Geometry check sheet. Reference: the model listing, model coordinates, mm. A direction names the side the tool comes from. Coordinates: 2 decimals unless noted, no trailing zeros. Loops run counter-clockwise (first coordinate to the right, second up) from the corner with the lowest first, then second, coordinate; pieces in that order, holes last. Notation, with made-up numbers: (17.5, 67) - (62.5, 67) arc R27 cw to (62.5, 95) - close; hole circle Ø1 at (-9.75, 52). An arc over 180 degrees is marked (long way). Write item = value, one per line. Start each with the question number.
from build123d import *

# Parameters (mm, degrees)
SZKIC1_W                    = 27
SZKIC1_H                    = 30
SZKIC1_R                    = 1.6
DODANIE_WYCI_GNI_CIE1_DEPTH = 2
DODANIE_WYCI_GNI_CIE2_DEPTH = 8
ZAOKR_GLENIE1_R             = 4
ZAOKR_GLENIE2_R             = 2


with BuildPart() as part:
    # Szkic1 → Dodanie-wyciągnięcie1 (new body)
    with BuildSketch(Plane(origin=(0, 0, 0), x_dir=(1, 0, 0), z_dir=(0, 1, 0))):
        Rectangle(SZKIC1_W, SZKIC1_H)
        with Locations(Location((10, 0, 0), (0, 0, 270))):
            Circle(SZKIC1_R, mode=Mode.SUBTRACT)
        with Locations(Location((-10, 0, 0), (0, 0, 270))):
            Circle(SZKIC1_R, mode=Mode.SUBTRACT)
    extrude(amount=DODANIE_WYCI_GNI_CIE1_DEPTH)

    # Szkic2 → Dodanie-wyciągnięcie2 (add)
    with BuildSketch(Plane.XZ):
        with BuildLine():
            Line((-13.5, 8), (-13.5, 15))
            Line((-13.5, 15), (-6.5, 15))
            ThreePointArc((-6.5, 15), (-8.550252532, 10.050252532), (-13.5, 8))
        make_face()
        with BuildLine():
            Line((13.5, 8), (13.5, 15))
            Line((13.5, 15), (6.5, 15))
            ThreePointArc((6.5, 15), (8.550252532, 10.050252532), (13.5, 8))
        make_face()
        with BuildLine():
            Line((13.5, -15), (6.5, -15))
            ThreePointArc((6.5, -15), (8.550252532, -10.050252532), (13.5, -8))
            Line((13.5, -8), (13.5, -15))
        make_face()
        with BuildLine():
            Line((-13.5, -8), (-13.5, -15))
            Line((-13.5, -15), (-6.5, -15))
            ThreePointArc((-6.5, -15), (-8.550252532, -10.050252532), (-13.5, -8))
        make_face()
    extrude(amount=DODANIE_WYCI_GNI_CIE2_DEPTH)

    # Zaokrąglenie1
    zaokr_glenie1_edges = [part.edges().sort_by_distance(p)[0] for p in [
        (13.5, -3, 15),
        (-13.5, -3, 15),
        (-13.5, -3, -15),
        (13.5, -3, -15),
    ]]
    fillet(zaokr_glenie1_edges, radius=ZAOKR_GLENIE1_R)

    # Zaokrąglenie2
    zaokr_glenie2_edges = [part.edges().sort_by_distance(p)[0] for p in [
        (-6.5, -4, 15),
        (-13.5, -4, 8),
        (6.5, -4, 15),
        (13.5, -4, 8),
        (13.5, -4, -8),
        (6.5, -4, -15),
        (-6.5, -4, -15),
        (-13.5, -4, -8),
    ]]
    fillet(zaokr_glenie2_edges, radius=ZAOKR_GLENIE2_R)


solid = part.part
(1) Scan lines: line 1 (X direction, y = 1.4, z = 0); line 2 (Y direction, x = 2, z = -5); line 3 (X direction, y = 1.5, z = -1). Record each from-to range of solid material in increasing order.
(2) Sectioned sample at B-B on z = 0. Enter the section's corners in (x, y), plus the area to 3 significant figures.
(3) Depth check by flat-ended pin: pin 1 (5 mm diameter, centred on x = 10, z = 0, fed in from -Y). Enter the tip coordinate at first touch or a pass-through.
(4) Sectioned sample at A-A on y = -2.5. Enter the section's corners in (x, z), plus the area to 3 significant figures.
(5) Draft check along X on faces 3 (the face through (-12.359, -3.07, -13.797)), 4 (the face through (-11.56, 0.99, -0.35)), 5 (the face through (0, 2, 0)), 6 (the face through (12.359, -3.07, -13.797)). Enter one of: pulls with the +X half, pulls with the -X half, needs draft (parallel to the pull), parting line crosses it, or undercut.
(6) Sectioned sample at D-D on x = 10. Enter the section's corners in (y, z), plus the area to 3 significant figures.
(7) Tool access check on faces 1 (the face through (8.5, -3.9, 10.1)), 2 (the face through (-0.7, 0.3, -15)). Record the directions out of +Z, -Z, +X, -X, +Y, -Y that give a thin tool (end or side, any length) a straight path to the whole face; none if there is none.
(8) Sectioned sample at C-C on y = 1.5. Enter the section's corners in (x, z), plus the area to 3 significant figures.
Working result:
q1.line_1 = -13.5 to -11.6, -8.4 to 8.4, 11.6 to 13.5
q1.line_2 = 0 to 2
q1.line_3 = -13.5 to -11.25, -8.75 to 8.75, 11.25 to 13.5
q2.outline = (-13.5, 0) - (-11.6, 0) - (-11.6, 2) - (-13.5, 2) - close; (-8.4, 0) - (8.4, 0) - (8.4, 2) - (-8.4, 2) - close; (11.6, 0) - (13.5, 0) - (13.5, 2) - (11.6, 2) - close
q2.area = 41.2 mm2
q3.pin_1 = 0
q4.outline = (-13.5, -11) arc R4 ccw to (-9.5, -15) - (-8.92, -15) arc R2 ccw to (-7.08, -12.2) arc R7 ccw to (-10.7, -8.58) arc R2 ccw to (-13.5, -10.42) - close; (-13.5, 10.42) arc R2 ccw to (-10.7, 8.58) arc R7 ccw to (-7.08, 12.2) arc R2 ccw to (-8.92, 15) - (-9.5, 15) arc R4 ccw to (-13.5, 11) - close; (7.08, -12.2) arc R2 ccw to (8.92, -15) - (9.5, -15) arc R4 ccw to (13.5, -11) - (13.5, -10.42) arc R2 ccw to (10.7, -8.58) arc R7 ccw to start; (7.08, 12.2) arc R7 ccw to (10.7, 8.58) arc R2 ccw to (13.5, 10.42) - (13.5, 11) arc R4 ccw to (9.5, 15) - (8.92, 15) arc R2 ccw to start
q4.area = 128 mm2
q5.face_3 = pulls with the -X half
q5.face_4 = undercut
q5.face_5 = needs draft
q5.face_6 = pulls with the +X half
q6.outline = (-8, -14.97) - (2, -14.97) - (2, -1.6) - (0, -1.6) - (0, -8.94) - (-8, -8.94) - close; (-8, 8.94) - (0, 8.94) - (0, 1.6) - (2, 1.6) - (2, 14.97) - (-8, 14.97) - close
q6.area = 150 mm2
q7.face_1 = -Y
q7.face_2 = -Z, +X, -X, +Y, -Y
q8.outline = (-13.5, -11) arc R4 ccw to (-9.5, -15) - (9.5, -15) arc R4 ccw to (13.5, -11) - (13.5, 11) arc R4 ccw to (9.5, 15) - (-9.5, 15) arc R4 ccw to (-13.5, 11) - close; hole circle Ø3.2 at (-10, 0); hole circle Ø3.2 at (10, 0)
q8.area = 780 mm2
